Geometry: see drawing. Coordinates: mm, zero at the bounding-box minimum. Coordinates: 2 decimals unless noted, no trailing zeros. Loops run counter-clockwise (first coordinate to the right, second up) from the corner with the lowest first, then second, coordinate; pieces in that order, holes last. Notation, with made-up numbers: (39.25, 21) -> (70.25, 21) arc R24 ccw to (70.25, 42) -> close; hole circle Ø6 at (16, 50.5). An arc over 180 degrees is marked (long way). One line per item, written item: value. Start each with the question number.
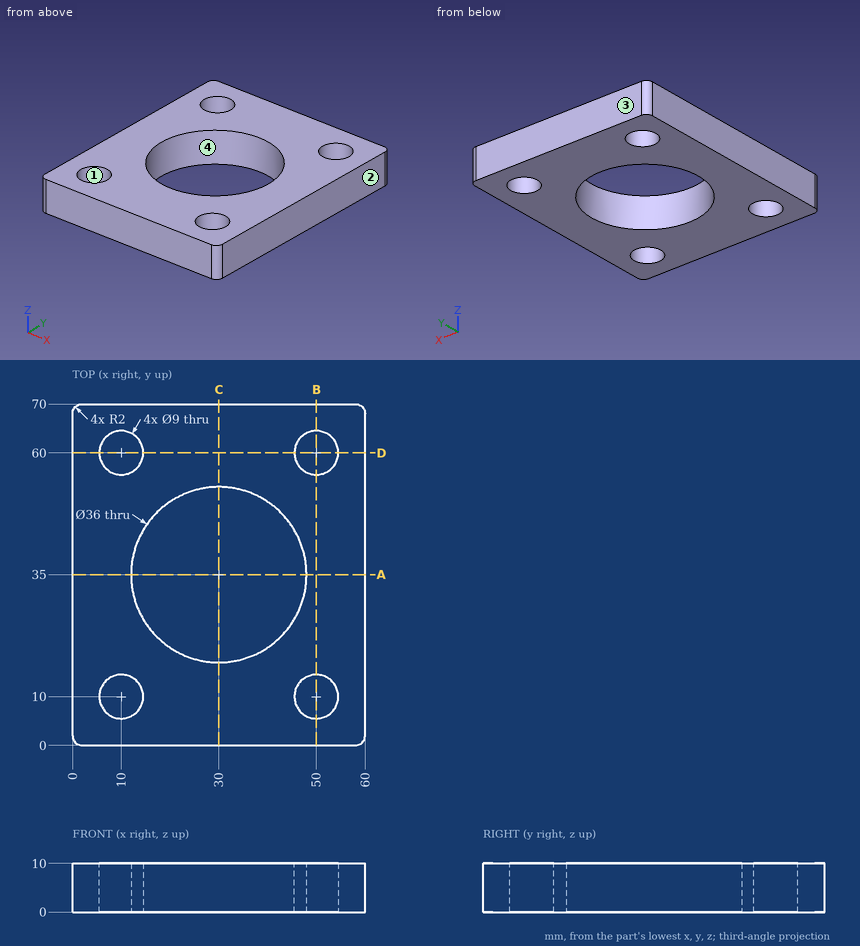
1. Section A-A on y = 35. Return the cut outline in (x, z), plus the area to 3 significant figures.
2. Pin query (flat end, axial travel): pin 1 Ø5.5 at (x, y) = (10, 10) entering from -Z. Return the tip coordinate at first contact, or that it passes through.
3. Section C-C on x = 30. Return the cut outline in (y, z), plus the area to 3 significant figures.
4. Section B-B on x = 50. Return the cut outline in (y, z).
5. Section D-D on y = 60. Return the cut outline in (x, z), plus the area to 3 significant figures.
6. Line query: L1, parallel to Y at x = 10, z = 4; L2, parallel to Y at x = 30, z = 4.5; L3, parallel to Y at x = 6.5, z = 8. Output: solid intervals per line, ascending. Write a range as [from, to].
7. Draft query along Y for the marked faces 1, 2, 3 and 4. Return one class per face: released by +Y, released by -Y, zero draft, split by the parting line, or undercut.
Checks:
1. outline: (0, 0) -> (12, 0) -> (12, 10) -> (0, 10) -> close; (48, 0) -> (60, 0) -> (60, 10) -> (48, 10) -> close
1. area: 240 mm²
2. pin 1: through
3. outline: (0, 0) -> (17, 0) -> (17, 10) -> (0, 10) -> close; (53, 0) -> (70, 0) -> (70, 10) -> (53, 10) -> close
3. area: 340 mm²
4. outline: (0, 0) -> (5.5, 0) -> (5.5, 10) -> (0, 10) -> close; (14.5, 0) -> (55.5, 0) -> (55.5, 10) -> (14.5, 10) -> close; (64.5, 0) -> (70, 0) -> (70, 10) -> (64.5, 10) -> close
5. outline: (0, 0) -> (5.5, 0) -> (5.5, 10) -> (0, 10) -> close; (14.5, 0) -> (45.5, 0) -> (45.5, 10) -> (14.5, 10) -> close; (54.5, 0) -> (60, 0) -> (60, 10) -> (54.5, 10) -> close
5. area: 420 mm²
6. L1: [0, 5.5], [14.5, 55.5], [64.5, 70]
6. L2: [0, 17], [53, 70]
6. L3: [0, 7.17], [12.83, 57.17], [62.83, 70]
7. face 1: undercut
7. face 2: zero draft
7. face 3: released by +Y
7. face 4: undercut
